Geometry: final body of the model. Coordinates: model frame, mm. A direction names the side the tool comes from. Give positions to 0.01 mm unless a question says otherwise; leave off trailing zeros. Loops run counter-clockwise (first coordinate to the right, second up) from the corner with the lowest first, then second, coordinate; pieces in that order, holes last. Notation, with made-up numbers: (-15, 69.25) -> (-3, 69.25) arc R20 ccw to (-3, 89.25) -> close; hole circle Ø9 at (43.25, 64). An arc over 180 degrees is marked (long way). Answer in a Markdown table with one row per item. Add a question column.
1) Section query D-D (z = 0). Give the number of separate pieces and of enclosed holes in the cut face, plus the area to 3 significant figures.
2) Line query: line 1 (Z direction, x = 41.75, y = 0); line 2 (X direction, y = 16.5, z = -33); line 3 (Z direction, x = 37, y = 17). Output: solid intervals per line, ascending. Write a range as from..to.
3) Section query A-A (z = 32). Return the cut outline in (x, y).
4) Section query B-B (x = 25). Return the cut outline in (y, z), plus the area to 3 significant figures.
5) Access query for faces 1 (the cylindrical face through (32.629, 23.846, 7.509)), 2 (the flat face through (48, -3, -8.2)), 3 (the cylindrical face through (45.887, -23.185, 5.149)). Directions: +Z, -Z, +X, -X, +Y, -Y. A direction counts if a zero-diameter tool reaches every point of the face in a straight line with its end or side. Return the directions, or none.
6) Draft query along X for faces 4 (the flat face through (0, 17, -17)), 5 (the flat face through (45, -9.1, -22.1)), 6 (the cylindrical face through (41.187, 0.676, 19.646)). Return one class per face: +X half, -X half, draft (parallel to the pull), parting line (faces both ways), or undercut.
7) First-contact query: P1, Ø2.5, axis at y = 32, z = 0, coming from the -X side; P2, Ø2, axis at x = 13, y = 13, coming from the +Z side; P3, Ø12, axis at x = 15, z = 11.5, coming from the +Y side; P4, Ø6, axis at y = 17.5, z = 0, coming from the -X side. Flat tips, straight axial feed; report the tip coordinate or a pass-through.
```python
from build123d import *

# Parameters (mm, degrees)
CSK_FOR_M4_FLAT_HEAD_MACHINE_SCREW1_D           = 4.5
CSK_FOR_M4_FLAT_HEAD_MACHINE_SCREW1_DEPTH       = 15
CSK_FOR_M4_FLAT_HEAD_MACHINE_SCREW1_CSINK_D     = 9.4
CSK_FOR_M4_FLAT_HEAD_MACHINE_SCREW1_CSINK_ANGLE = 90
FILLET1_R                                       = 0.6
SKETCH9_R                                       = 25
SKETCH9_R_2                                     = 23.75
CUT_EXTRUDE1_DEPTH                              = 1.8
M4_CLEARANCE_HOLE1_D                            = 4.5
M4_CLEARANCE_HOLE1_DEPTH                        = 2.5


with BuildPart() as part:
    # Sketch2 → Revolve1 (revolve)
    with BuildSketch(Plane.XY):
        Polygon((0, 21), (35, 21), (35, 12.5), (48, 12.5), (48, 8.5), (50, 8.5), (50, 25), (20, 25), (20, 26), (2.5, 26), (2.5, 39), (0, 39), (0, 26), align=None)
    revolve(axis=Axis((-64.103352454, 0, 0), (1, 0, 0)))

    # CSK for M4 Flat Head Machine Screw1
    with Locations(Plane(origin=(50, 0, 0), x_dir=(0, 0, -1), z_dir=(1, 0, 0))):
        with Locations((0, 17.5), (17.5, 0), (0, -17.5), (-17.5, 0)):
            CounterSinkHole(CSK_FOR_M4_FLAT_HEAD_MACHINE_SCREW1_D / 2, CSK_FOR_M4_FLAT_HEAD_MACHINE_SCREW1_CSINK_D / 2, depth=CSK_FOR_M4_FLAT_HEAD_MACHINE_SCREW1_DEPTH, counter_sink_angle=CSK_FOR_M4_FLAT_HEAD_MACHINE_SCREW1_CSINK_ANGLE)

    # Fillet1
    fillet1_edges = [part.edges().sort_by_distance(p)[0] for p in [
        (20, -25, 0),
    ]]
    fillet(fillet1_edges, radius=FILLET1_R)

    # Sketch9 → Cut-Extrude1 (cut)
    with BuildSketch(Plane(origin=(45, 0, 0), x_dir=(0, 0, -1), z_dir=(1, 0, 0))):
        Circle(SKETCH9_R)
        Circle(SKETCH9_R_2, mode=Mode.SUBTRACT)
    extrude(amount=CUT_EXTRUDE1_DEPTH, mode=Mode.SUBTRACT)

    # M4 Clearance Hole1
    with Locations(Plane.ZY):
        with Locations((0, 32), (0, -32), (32, 0), (-32, 0)):
            Hole(M4_CLEARANCE_HOLE1_D / 2, depth=M4_CLEARANCE_HOLE1_DEPTH)


solid = part.part
```
Evaluation:
| question | item | result |
|---|---|---|
| 1 | separate pieces | 6 |
| 1 | enclosed holes | 0 |
| 1 | area | 602 mm² |
| 2 | line 1 | -25..-19.75, -15.25..-12.5, 12.5..15.25, 19.75..25 |
| 2 | line 2 | 0..2.5 |
| 2 | line 3 | -18.33..-2.19, 2.19..18.33 |
| 3 | outline | (0, -22.29) -> (2.5, -22.29) -> (2.5, -2.25) -> (0, -2.25) -> close; (0, 2.25) -> (2.5, 2.25) -> (2.5, 22.29) -> (0, 22.29) -> close |
| 4 | outline | circle Ø50 at (0, 0); hole circle Ø42 at (0, 0) |
| 4 | area | 578 mm² |
| 5 | face 1 | +X |
| 5 | face 2 | -X |
| 5 | face 3 | none |
| 6 | face 4 | -X half |
| 6 | face 5 | undercut |
| 6 | face 6 | draft |
| 7 | P1 | through |
| 7 | P2 | z = 23.07 |
| 7 | P3 | y = 25.41 |
| 7 | P4 | x = 35 |
